```python
from build123d import *

# Parameters (mm, degrees)
ESQUISSE1_R        = 14.059058324
ESQUISSE1_R_2      = 13.059058324
BOSS_EXTRU_3_DEPTH = 100
ESQUISSE1_6_R      = 17.059058324
ESQUISSE1_6_R_2    = 14.059058324
BOSS_EXTRU_4_DEPTH = 5
BOSS_EXTRU_5_START = -5
ESQUISSE2_R        = 17.059058324
ESQUISSE2_R_2      = 14.059058324
BOSS_EXTRU_5_DEPTH = 5


with BuildPart() as part:
    # Esquisse1 → Boss.-Extru.3 (new body)
    with BuildSketch(Plane.XY):
        Circle(ESQUISSE1_R)
        Circle(ESQUISSE1_R_2, mode=Mode.SUBTRACT)
    extrude(amount=BOSS_EXTRU_3_DEPTH)

    # Esquisse1<6> → Boss.-Extru.4 (add)
    with BuildSketch(Plane.XY):
        Circle(ESQUISSE1_6_R)
        Circle(ESQUISSE1_6_R_2, mode=Mode.SUBTRACT)
    extrude(amount=BOSS_EXTRU_4_DEPTH)

    # Esquisse2 → Boss.-Extru.5 (add)
    with BuildSketch(Plane.XY.offset(100).offset(BOSS_EXTRU_5_START)):
        Circle(ESQUISSE2_R)
        Circle(ESQUISSE2_R_2, mode=Mode.SUBTRACT)
    extrude(amount=BOSS_EXTRU_5_DEPTH)


solid = part.part
```
Source: CAD feature listing. Evaluate the final solid. Frame: model axes, mm. A direction names the side the tool comes from. Give positions to 0.01 mm unless a question says otherwise; leave off trailing zeros. Write each loop counter-clockwise with the first axis right and the second up, starting at its lowest first coordinate (ties: lowest second). Pieces come first, ordered by that corner, then holes.
1. Section query A-A (y = 0). Return the cut outline in (x, z).
2. Material intervals for line 1 along Z through (x, y) = (9.5, -14); line 2 along Y through (x, z) = (0, 29); line 3 along X through (y, z) = (-9.5, 59.5), sorted ascending.
3. First-contact query: pin 1 (1 mm diameter, centred on y = -4.5, z = 85, fed in from -X); pin 2 (1 mm diameter, centred on x = -0.5, z = 41, fed in from +Y); pin 3 (6 mm diameter, centred on y = -1.5, z = 77, fed in from -X). Flat tips, straight axial feed; report the tip coordinate or a pass-through.
4. Pull-direction query (X, two-part tool) for faces 1 (the face through (-4, -13, 100)), 2 (the face through (-3.698, -16.653, 2.465)), 3 (the face through (-1.7, 12.948, 49.3)); classes: +X half, -X half, draft (parallel to the pull), parting line (faces both ways), or undercut.
5. Access query for faces 4 (the face through (-11.16, -8.55, 49.37)), 5 (the face through (-3.698, -16.653, 97.465)). Directions: +Z, -Z, +X, -X, +Y, -Y. A direction counts if a zero-diameter tool reaches every point of the face in a straight line with its end or side. Return the directions, or none.
6. Section query C-C (z = 32.5). Return the cut outline in (x, y).
Output values:
1. outline: (-17.06, 0) - (-13.06, 0) - (-13.06, 100) - (-17.06, 100) - (-17.06, 95) - (-14.06, 95) - (-14.06, 5) - (-17.06, 5) - close; (13.06, 0) - (17.06, 0) - (17.06, 5) - (14.06, 5) - (14.06, 95) - (17.06, 95) - (17.06, 100) - (13.06, 100) - close
2. line 1: z = 0 to 5, 95 to 100
2. line 2: y = -14.06 to -13.06, 13.06 to 14.06
2. line 3: x = -10.36 to -8.96, 8.96 to 10.36
3. pin 1: stops at x = -13.48
3. pin 2: stops at y = 14.06
3. pin 3: stops at x = -14.06
4. face 1: draft
4. face 2: parting line
4. face 3: undercut
5. face 4: none
5. face 5: +Z, -Z
6. outline: circle Ø28.12 at (0, 0); hole circle Ø26.12 at (0, 0)
